Verification items for the finished model (mm, model axes). A direction names the side the tool comes from. Give positions to 0.01 mm unless a question says otherwise; leave off trailing zeros. Loops run counter-clockwise (first coordinate to the right, second up) from the corner with the lowest first, then second, coordinate; pieces in that order, holes last. Notation, with made-up numbers: M 79.5,-6.75 L 136.5,-6.75 A20 ccw 136.5,-1.75 Z; hole C 5,81 d1. An arc over 180 degrees is marked long. Put each result on its own line as item: value. Start each with the question number.
from build123d import *

# Parameters (mm, degrees)
BOSS_EXTRUDE1_DEPTH = 30
SKETCH2_R           = 2
CUT_EXTRUDE1_DEPTH  = 7
FILLET1_R           = 10
FILLET2_R           = 5
BOSS_EXTRUDE2_START = 15
SKETCH3_W           = 30
SKETCH3_H           = 30
SKETCH3_W_2         = 18.5
SKETCH3_H_2         = 18.5
BOSS_EXTRUDE2_DEPTH = 25
FILLET3_R           = 20
SKETCH4_R           = 2
CUT_EXTRUDE2_DEPTH  = 30


with BuildPart() as part:
    # Sketch1 → Boss-Extrude1 (new body)
    with BuildSketch(Plane(origin=(0, 0, 0), x_dir=(1, 0, 0), z_dir=(0, 1, 0))):
        with BuildLine():
            ThreePointArc((-24.171263931, 4), (0, 24.5), (24.171263931, 4))
            Line((24.171263931, 4), (49.171263931, 4))
            Line((49.171263931, 4), (49.171263931, 10))
            Line((49.171263931, 10), (30.397368307, 10))
            ThreePointArc((30.397368307, 10), (0, 32), (-30.397368307, 10))
            Line((-30.397368307, 10), (-49.171263931, 10))
            Line((-49.171263931, 10), (-49.171263931, 4))
            Line((-49.171263931, 4), (-24.171263931, 4))
        make_face()
    extrude(amount=BOSS_EXTRUDE1_DEPTH)

    # Sketch2 → Cut-Extrude1 (cut, through all)
    with BuildSketch(Plane(origin=(0, 0, -10), x_dir=(-1, 0, 0), z_dir=(0, 0, -1))):
        with Locations((-39.171263931, 22)):
            Circle(SKETCH2_R)
        with Locations((-39.171263931, 8)):
            Circle(SKETCH2_R)
        with Locations((39.171263931, 8)):
            Circle(SKETCH2_R)
        with Locations((39.171263931, 22)):
            Circle(SKETCH2_R)
    extrude(amount=-CUT_EXTRUDE1_DEPTH, mode=Mode.SUBTRACT)

    # Fillet1
    fillet1_edges = [part.edges().sort_by_distance(p)[0] for p in [
        (-30.397368307, 15, -10),
        (30.397368307, 15, -10),
    ]]
    fillet(fillet1_edges, radius=FILLET1_R)

    # Fillet2
    fillet2_edges = [part.edges().sort_by_distance(p)[0] for p in [
        (-24.171263931, 15, -4),
        (24.171263931, 15, -4),
    ]]
    fillet(fillet2_edges, radius=FILLET2_R)

    # Sketch3 → Boss-Extrude2 (add)
    with BuildSketch(Plane(origin=(0, 0, -10), x_dir=(-1, 0, 0), z_dir=(0, 0, -1)).offset(BOSS_EXTRUDE2_START)):
        with Locations((0, 15)):
            Rectangle(SKETCH3_W, SKETCH3_H)
        with Locations((0, 15)):
            Rectangle(SKETCH3_W_2, SKETCH3_H_2, mode=Mode.SUBTRACT)
    extrude(amount=BOSS_EXTRUDE2_DEPTH)

    # Fillet3
    fillet3_edges = [part.edges().sort_by_distance(p)[0] for p in [
        (-15, 15, -28.26658805),
        (15, 15, -28.26658805),
    ]]
    fillet(fillet3_edges, radius=FILLET3_R)

    # Sketch4 → Cut-Extrude2 (cut)
    with BuildSketch(Plane(origin=(15, 0, 0), x_dir=(0, 0, -1), z_dir=(1, 0, 0))):
        with Locations((42, 15)):
            Circle(SKETCH4_R)
    extrude(amount=-CUT_EXTRUDE2_DEPTH, mode=Mode.SUBTRACT)


solid = part.part
Q1. Cross-section at B-B, the plane z = -42. Record the boundary of the cut face in (x, y).
Q2. Go/stop test with flat-tipped pins: pin 1 (5 mm diameter, centred on y = 15, z = -42, fed in from -X); pin 2 (2 mm diameter, centred on y = 7.5, z = -27, fed in from -X); pin 3 (3.5 mm diameter, centred on y = 19.5, z = -46, fed in from +X). Record where each tip stops, or that it passes through.
Q3. Cross-section at A-A, the plane y = 15. State how many separate pieces and enclosed holes the cut face has, then the cut area to 3 significant figures.
Q4. Set-up check for faces 4 (the face through (-43, 15, -10)), 5 (the face through (-9.25, 13, -40)), 6 (the face through (25.24, 14.79, -19.67)), 7 (the face through (25.182, 15.21, -4.935)): record each of +Z, -Z, +X, -X, +Y, -Y from which the full face is reachable in a straight line by a thin tool's end or side.
Q5. Scan lines: L1, parallel to X at y = 8.5, z = -40; L2, parallel to Y at x = -12.6, z = -42; L3, parallel to X at y = 20.75, z = -7.5. Record each from-to range of solid material in increasing order.
Q6. Cross-section at D-D, the plane x = 40. Record the boundary of the cut face in (y, z), then the cut area to 3 significant figures.
Q7. Release check for a two-part mould opening along Y. For faces 1 (the face through (0, 0, -25)), 2 (the face through (9.25, 13, -40)), 3 (the face through (43, 15, -10)) record: pulls with the +Y half, pulls with the -Y half, needs draft (parallel to the pull), parting line crosses it, or undercut.
Ans:
1. outline: M -15,0 L 15,0 L 15,13 L 9.25,13 L 9.25,5.75 L -9.25,5.75 L -9.25,13 L -15,13 Z; M -15,17 L -9.25,17 L -9.25,24.25 L 9.25,24.25 L 9.25,17 L 15,17 L 15,30 L -15,30 Z
2. pin 1: stops at x = -15
2. pin 2: stops at x = -19.35
2. pin 3: stops at x = 15
3. separate pieces: 3
3. enclosed holes: 0
3. area: 1,050 mm^2
4. face 4: -Z, -X, +Y, -Y
4. face 5: -Z
4. face 6: -Z, +X, +Y, -Y
4. face 7: +Z, +Y, -Y
5. L1: x = -15 to -9.25, 9.25 to 15
5. L2: y = 0 to 13, 17 to 30
5. L3: x = -49.17 to -40.73, -37.61 to -23.32, 23.32 to 37.61, 40.73 to 49.17
6. outline: M 0,-10 L 6.18,-10 L 6.18,-4 L 0,-4 Z; M 9.82,-10 L 20.18,-10 L 20.18,-4 L 9.82,-4 Z; M 23.82,-10 L 30,-10 L 30,-4 L 23.82,-4 Z
6. area: 136 mm^2
7. face 1: pulls with the -Y half
7. face 2: undercut
7. face 3: needs draft
